Verification items for the finished model (mm, model axes). Face numbers are marked on the shaded views. A direction names the side the tool comes from. Give positions to 0.01 mm unless a question says otherwise; leave off trailing zeros. Write each loop counter-clockwise with the first axis right and the second up, starting at its lowest first coordinate (ties: lowest second). Pieces come first, ordered by that corner, then holes. Notation, with made-up numbers: (25, -15) -> (55, -15) arc R32 cw to (55, 11) -> close; hole circle Ø4 at (12.25, -3.5). An arc over 180 degrees is marked (long way). Answer as CSV lines item,"result".
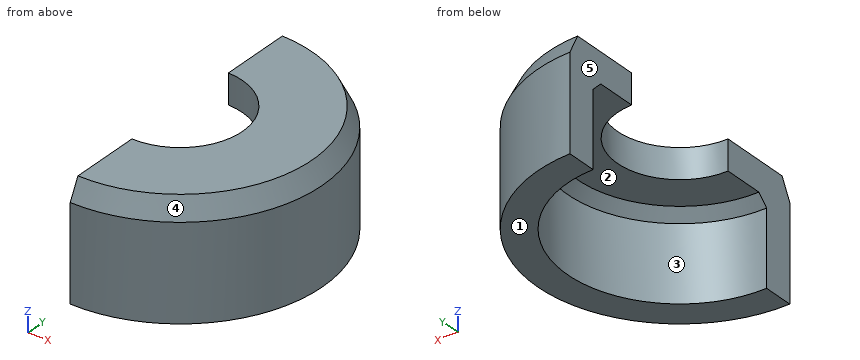
Autodesk Fusion 360 part; units mm, degrees
sketch "Sketch1" plane through (0, 0, 0) normal (1, 0, 0) x (0, 1, 0)
  line L0 (0, 0) -> (-26.3359, 0) construction
  line L1 (-11.25, 0) -> (-11.25, 8.5)
  line L2 (-11.25, 8.5) -> (-6.25, 8.5)
  line L3 (-11.25, 0) -> (-14.25, 0)
  line L4 (-14.25, 0) -> (-14.25, 11.5)
  line L5 (-14.25, 11.5) -> (-6.25, 11.5)
  line L6 (-6.25, 11.5) -> (-6.25, 8.5)
  line L7 (0, 0) -> (0, 80.4746)
  dimension "d1" = 8.5
  dimension "d3" = 22.5
  dimension "d4" = 12.5
  dimension "d5" = 3
  dimension "d6" = 3
revolve "Revolve1" add sketch "Sketch1" angle 180 about axis through (0, 0, 0) along (0, 0, 1)
chamfer "Chamfer1" distance 1 distance2 2 1 edges at (14.25, 0, 11.5) measured on face at (2.7221, 11.2267, 11.5)
chamfer "Chamfer2" distance 1 distance2 1 1 edges at (11.25, 0, 8.5) measured on face at (7.2314, 8.618, 5.6667)
equation "d6 = d5"
1) Section check A-A (y = 0). Record the boundary of the cut face in (x, z), and give its area (3 significant figures).
Reported:
outline,"(6.25, 8.5) -> (10.25, 8.5) -> (11.25, 7.5) -> (11.25, 0) -> (14.25, 0) -> (14.25, 9.5) -> (13.25, 11.5) -> (6.25, 11.5) -> close"
area,"49.0 mm²"
2) Scan lines: line 1 along Z through (x, y) = (9.25, -1.25); line 2 along Y through (x, z) = (5.5, 5.5); line 3 along Y through (x, z) = (10, 3). Record each from-to range of solid material in increasing order.
Reported:
line 1,"8.5 to 11.5"
line 2,"-13.15 to -9.81, 9.81 to 13.15"
line 3,"-10.15 to -5.15, 5.15 to 10.15"
3) Section check B-B (z = 7). Record the boundary of the cut face in (x, y), and give its area (3 significant figures).
Reported:
outline,"(0, -14.25) arc R14.25 ccw to (0, 14.25) -> (0, 11.25) arc R11.25 cw to (0, -11.25) -> close"
area,"120 mm²"
4) Draft check along Y on the marked faces 3, 4 and 5. Enter one of: +Y half, -Y half, draft (parallel to the pull), parting line (faces both ways), or undercut.
Reported:
face 3,"undercut"
face 4,"parting line"
face 5,"draft"
5) Depth check by flat-ended pin: pin 1 (1 mm diameter, centred on x = 9.5, y = 3.5, fed in from -Z); pin 2 (1 mm diameter, centred on y = -11, z = 3.5, fed in from +X); pin 3 (2 mm diameter, centred on y = 11, z = 9.5, fed in from -X); pin 4 (1.5 mm diameter, centred on x = 6.5, z = 8, fed in from -Y). Enter the tip coordinate at first touch or a pass-through.
Reported:
pin 1,"z = 8.13"
pin 2,"x = 9.63"
pin 3,"x = 0"
pin 4,"y = -13.04"
6) Tool access check on the marked faces 1 and 2. Record the directions out of +Z, -Z, +X, -X, +Y, -Y that give a thin tool (end or side, any length) a straight path to the whole face; none if there is none.
Reported:
face 1,"-Z, +X, -X, +Y, -Y"
face 2,"-Z, -X"
